Here's how the part is built. I have some questions about the finished solid (model axes, mm). Round coordinates to 2 decimals unless told otherwise and drop trailing zeros. Loops run counter-clockwise (first coordinate to the right, second up) from the corner with the lowest first, then second, coordinate; pieces in that order, holes last. Notation, with made-up numbers: M 84,23 L 138,23 A10 ccw 138,28 Z; hole C 62.25,69 d10. An arc over 180 degrees is marked long. Answer as a JSON object with one key per item and string values.
from build123d import *

# Parameters (mm, degrees)
SKETCH1_W                = 83.98
SKETCH1_H                = 147.35
PLATFORM_THICKNESS_DEPTH = 5
SKETCH2_R                = 10
IO_HOLE_1_DEPTH          = 170.675168778
SKETCH3_R                = 1.1
MOUNTING_HOLES_DEPTH     = 170.675168778


with BuildPart() as part:
    # Sketch1 → platform_thickness (new body)
    with BuildSketch(Plane.XY):
        with Locations((-41.99, 73.675)):
            Rectangle(SKETCH1_W, SKETCH1_H)
    extrude(amount=PLATFORM_THICKNESS_DEPTH)

    # Sketch2 → io_hole_1 (cut, through all)
    with BuildSketch(Plane(origin=(0, 0, 0), x_dir=(-1, 0, 0), z_dir=(0, 0, -1))):
        with Locations((41.99, 100.585)):
            Circle(SKETCH2_R)
        with Locations((41.99, 46.765)):
            Circle(SKETCH2_R)
    extrude(amount=-IO_HOLE_1_DEPTH, mode=Mode.SUBTRACT)

    # Sketch3 → mounting_holes (cut, through all)
    with BuildSketch(Plane(origin=(0, 0, 0), x_dir=(-1, 0, 0), z_dir=(0, 0, -1))):
        with Locations((2.5, 144.85)):
            Circle(SKETCH3_R)
        with Locations((81.48, 144.85)):
            Circle(SKETCH3_R)
        with Locations((81.48, 2.5)):
            Circle(SKETCH3_R)
        with Locations((2.5, 2.5)):
            Circle(SKETCH3_R)
    extrude(amount=-MOUNTING_HOLES_DEPTH, mode=Mode.SUBTRACT)


solid = part.part
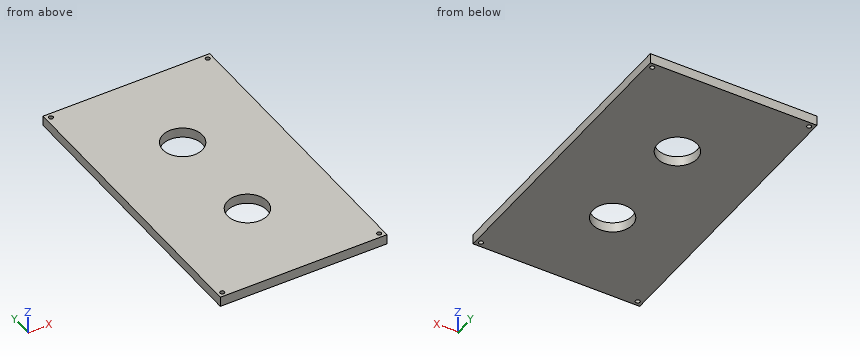
Item 1: I want a section at A-A on x = -41.99. List the corners of the cut face in (y, z) for me (3 decimals), plus the area to 3 significant figures.
Solution:
{"outline": "M 0,0 L 36.765,0 L 36.765,5 L 0,5 Z; M 56.765,0 L 90.585,0 L 90.585,5 L 56.765,5 Z; M 110.585,0 L 147.35,0 L 147.35,5 L 110.585,5 Z", "area": "537 mm2"}
Item 2: I want a section at B-B on z = 3.55. List the corners of the cut face in (x, y) for me (3 decimals), plus the area to 3 significant figures.
Solution:
{"outline": "M -83.98,0 L 0,0 L 0,147.35 L -83.98,147.35 Z; hole C -81.48,2.5 d2.2; hole C -81.48,144.85 d2.2; hole C -41.99,46.765 d20; hole C -41.99,100.585 d20; hole C -2.5,2.5 d2.2; hole C -2.5,144.85 d2.2", "area": "11,700 mm2"}
Item 3: If I drill on L1, parallel to Y at x = -41.99, z = 3.95 (3 decimals); L2, parallel to X at y = 144.85, z = 2.5; L3, parallel to Y at x = -2.5, z = 2.15, over which ranges is the centre line in solid material (lowest first)? Write a range as from..to.
Solution:
{"L1": "y = 0..36.765, 56.765..90.585, 110.585..147.35", "L2": "x = -83.98..-82.58, -80.38..-3.6, -1.4..0", "L3": "y = 0..1.4, 3.6..143.75, 145.95..147.35"}
